Check sheet for the drawn part. Datum: minimum x, y, z corner. Units: mm. A direction names the side the tool comes from. Give positions to 0.01 mm unless a question says otherwise; leave off trailing zeros. Write each loop counter-clockwise with the first axis right and the second up, starting at its lowest first coordinate (ties: lowest second). Pieces come first, ordered by that corner, then holes. Notation, with made-up numbers: (64.5, 23) - (95.5, 23) arc R33 ccw to (95.5, 62) - close; hole circle Ø9 at (-21.5, -33). An arc over 180 degrees is marked (long way). Answer as a JSON object with one key per item and string values. Group by question number.
Item 1: Scan lines: line 1 along X through (y, z) = (1.25, 0.5); line 2 along Y through (x, z) = (15.5, 2); line 3 along Z through (x, y) = (10, 10.5). Record each from-to range of solid material in increasing order. Write a range as [from, to].
Item 2: Go/stop test with flat-tipped pins: pin 1 (1.5 mm diameter, centred on x = 5, z = 3, fed in from -Y); pin 2 (0.8 mm diameter, centred on y = 1.5, z = 4, fed in from +X). Record where each tip stops, or that it passes through.
Item 3: Draft check along X on the marked faces 1, 2 and 3. Enter one of: +X half, -X half, draft (parallel to the pull), parting line (faces both ways), or undercut.
Item 4: Sectioned sample at C-C, the plane z = 3.75. Record the boundary of the cut face in (x, y), and give its area (3 significant figures).
Item 5: Tool access check on the marked faces 4, 5 and 6. Record the directions out of +Z, -Z, +X, -X, +Y, -Y that give a thin tool (end or side, any length) a straight path to the whole face; none if there is none.
Item 6: Sectioned sample at A-A, the plane y = 1.5. Record the boundary of the cut face in (x, z).
Item 7: Sectioned sample at B-B, the plane x = 14.5. Record the boundary of the cut face in (y, z).
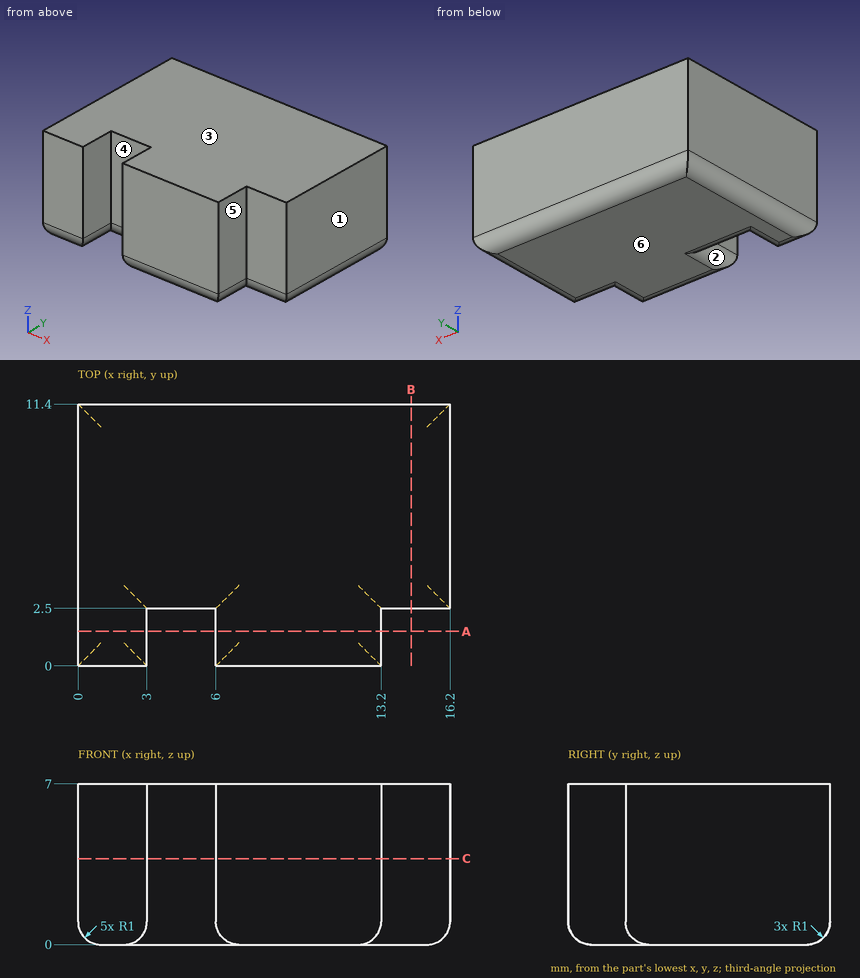
Geometry check:
{
 "1": {"line 1": "[0.13, 2.87], [6.13, 13.07]", "line 2": "[2.5, 11.4]", "line 3": "[0.01, 7]"},
 "2": {"pin 1": "y = 2.5", "pin 2": "x = 13.2"},
 "3": {"face 1": "+X half", "face 2": "undercut", "face 3": "draft"},
 "4": {"outline": "(0, 0) - (3, 0) - (3, 2.5) - (6, 2.5) - (6, 0) - (13.2, 0) - (13.2, 2.5) - (16.2, 2.5) - (16.2, 11.4) - (0, 11.4) - close", "area": "170 mm^2"},
 "5": {"face 4": "+Z, -Z, -Y", "face 5": "+Z, -Z, +X, -Y", "face 6": "-Z, +X, -X, +Y, -Y"},
 "6": {"outline": "(0, 1) arc R1 ccw to (1, 0) - (2, 0) arc R1 ccw to (3, 1) - (3, 7) - (0, 7) - close; (6, 1) arc R1 ccw to (7, 0) - (12.2, 0) arc R1 ccw to (13.2, 1) - (13.2, 7) - (6, 7) - close"},
 "7": {"outline": "(2.5, 1) arc R1 ccw to (3.5, 0) - (10.4, 0) arc R1 ccw to (11.4, 1) - (11.4, 7) - (2.5, 7) - close"}
}
